from build123d import *

# Parameters (mm, degrees)
F0_R        = 1.5875
F1_DEPTH    = 1.5875
F2_T1_DEPTH = 5.9319428422


# Not quite as in the source:
# - a fillet or chamfer that OpenCascade refuses, or shapes differently, is made with other operations: its cross-section is extruded or revolved along the edge and cut away or added


with BuildPart() as f1:
    # F0 (on Front) → F1 (new body, symmetric)
    with BuildSketch(Plane.XZ):
        with BuildLine():
            ThreePointArc((3.7381009291, -0.0336915449), (4.4820497049, 1.7623596793), (6.2781009291, 2.5063084551))
            Line((6.2781009291, 2.5063084551), (9.3939231872, 2.5063084551))
            ThreePointArc((9.3939231872, 2.5063084551), (-2.459861222, 12.0150971251), (-8.3760311943, -1.9823383417))
            Line((-8.3760311943, -1.9823383417), (-7.3443697718, -1.3867083417))
            Line((-7.3443697718, -1.3867083417), (-5.0381606197, -5.381179766))
            ThreePointArc((-5.0381606197, -5.381179766), (-0.7165786385, -6.7265825886), (3.7381009291, -5.9253276194))
            Line((3.7381009291, -5.9253276194), (3.7381009291, -0.0336915449))
        make_face()
        with Locations((-0.1472348195, 2.7336615811)):
            Circle(F0_R, mode=Mode.SUBTRACT)
    extrude(amount=F1_DEPTH, both=True)

    # F2: chamfer of 0.508 on 1 edges, made by hand

    # F2_s2 → F2_t1 (cut)
    with BuildSketch(Plane.XZ.offset(-2.9659714211)):
        with BuildLine():
            Line((-7.9236877385, -1.7211777257), (-8.6312397675, -1.5100480025))
            ThreePointArc((-8.6312397675, -1.5100480025), (-8.5103751964, -1.7416719985), (-8.3760311943, -1.9823383417))
            Line((-8.3760311943, -1.9823383417), (-7.9236877385, -1.7211777257))
        make_face()
    extrude(amount=F2_T1_DEPTH, mode=Mode.SUBTRACT)


solid = f1.part
For this review, take the finished solid that the model builds, in its own axes (mm). A direction names the side the tool comes from. Coordinates: 2 decimals unless noted, no trailing zeros. Order: outer loops, then holes, each group sorted by start corner. A loop starts at its lowest first (then second) coordinate and runs counter-clockwise, first axis right, second up. Notation, with made-up numbers: (86, 83.25) -> (91, 83.25) arc R13 cw to (91, 88.25) -> close; hole circle Ø1 at (-18.75, 85.5). An arc over 180 degrees is marked (long way). Return JSON: item names as keys, results as strings.
1. The part is to be moulded in two halves that separate along Z. For faces 3 (the flat face through (-6.207, -0.022, -3.356)), 4 (the cylindrical face through (-1.961, -0.022, 12.127)), 5 (the cylindrical face through (-0.491, 0.022, 1.184)), say which applies: +Z half, -Z half, draft (parallel to the pull), parting line (faces both ways), or undercut.
Answer block:
{"face 3": "-Z half", "face 4": "parting line", "face 5": "undercut"}
2. We need section A-A on x = -0.5. Write out the cut boundary in (y, z).
Answer block:
{"outline": "(-1.59, -6.74) -> (1.59, -6.74) -> (1.59, 1.19) -> (-1.59, 1.19) -> close; (-1.59, 4.28) -> (1.59, 4.28) -> (1.59, 12.3) -> (-1.59, 12.3) -> close"}
3. For line 1 (Z direction, x = -0.25, y = 1); line 2 (Z direction, x = 0, y = -1.15); line 3 (Z direction, x = 7.5, y = -0.75), list the stretches that pass through material, from the lowest coordinate up. Write a range as from..to.
Answer block:
{"line 1": "-6.74..1.15, 4.32..12.3", "line 2": "-6.74..1.15, 4.31..12.3", "line 3": "2.51..8.49"}
4. For pin 1 Ø1 at (y, z) = (-0.5, 8) entering from +X, flat-tipped, find the tip position at first contact; note if it passes through.
Answer block:
{"pin 1": "x = 8.15"}
5. We need section D-D on x = 5.25. Write out the cut boundary in (y, z), and give its area (3 significant figures).
Answer block:
{"outline": "(-1.59, 2.29) -> (1.59, 2.29) -> (1.59, 10.64) -> (-1.59, 10.64) -> close", "area": "26.5 mm²"}
6. We need section C-C on z = 5.5. Write out the cut boundary in (x, y), and give its area (3 significant figures).
Answer block:
{"outline": "(-9.26, -1.59) -> (9, -1.59) -> (9, 1.59) -> (-9.26, 1.59) -> close", "area": "58.0 mm²"}
7. Machinability: for faces 1 (the cylindrical face through (-0.78, -0.022, -6.722)), 2 (the flat face through (3.738, 0, -3)), which of the approach directions +Z, -Z, +X, -X, +Y, -Y give a long, thin tool a straight path to every point of the face, cutting with its end or side? Answer none if there is none.
Answer block:
{"face 1": "-Z, +Y, -Y", "face 2": "-Z, +X, +Y, -Y"}
